Could you check a few things on this model? Use its own coordinates, in mm. Round coordinates to 2 decimals unless told otherwise and drop trailing zeros. Loops run counter-clockwise (first coordinate to the right, second up) from the corner with the lowest first, then second, coordinate; pieces in that order, holes last. Notation, with made-up numbers: (1, -19.5) - (23, -19.5) arc R15 cw to (23, -5.5) - close; hole circle Ø11 at (65, -13). An arc over 180 degrees is marked (long way). Use one line per item in the form item = value.
```python
from build123d import *

# Parameters (mm, degrees)
SKETCH1_R               = 12.5
SKETCH1_R_2             = 3.5
BOSS_EXTRUDE1_DEPTH     = 12
CUT_EXTRUDE1_DEPTH      = 22
CUT_EXTRUDE1_DEPTH_BACK = 22
SKETCH2_R               = 12.5
FILLET2_R               = 1


with BuildPart() as part:
    # Sketch1 → Boss-Extrude1 (new body)
    with BuildSketch(Plane(origin=(0, 0, 0), x_dir=(1, 0, 0), z_dir=(0, 1, 0))):
        with Locations(Location((0, 0, 0), (0, 0, 270))):
            Circle(SKETCH1_R)
        with Locations(Location((0, 0, 0), (0, 0, 270))):
            Circle(SKETCH1_R_2, mode=Mode.SUBTRACT)
    extrude(amount=BOSS_EXTRUDE1_DEPTH)

    # Sketch2 → Cut-Extrude1 (cut, two sides: drawn at the far end of the back side and taken through both)
    with BuildSketch(Plane.XY.offset(-CUT_EXTRUDE1_DEPTH_BACK)):
        with Locations((0, 17)):
            Circle(SKETCH2_R)
    extrude(amount=CUT_EXTRUDE1_DEPTH + CUT_EXTRUDE1_DEPTH_BACK, mode=Mode.SUBTRACT)

    # Fillet2
    fillet2_edges = [part.edges().sort_by_distance(p)[0] for p in [
        (11.456439237, 12, 0),
        (-11.456439237, 12, 0),
    ]]
    fillet(fillet2_edges, radius=FILLET2_R)


solid = part.part
```
1. If we section it at D-D, the plane y = 1: Write out the boundary of the cut face in (x, z).
Solution:
outline = circle Ø25 at (0, 0); hole circle Ø7 at (0, 0)
2. If we section it at C-C, the plane y = 9.5: Write out the boundary of the cut face in (x, z), plus the area to 3 significant figures.
Solution:
outline = (-10, -7.5) - (-10, 7.5) arc R12.5 ccw to start; (10, -7.5) arc R12.5 ccw to (10, 7.5) - close
area = 51.1 mm^2
3. We'd pull the mould along X, two halves only. Please class faces 1 (the face through (-3, 0, 3)), 2 (the face through (2.86, 4.83, 2.6)), 3 (the face through (3.755, 4.583, 11.923)), 4 (the face through (3.47, 2.47, -0.46)): +X half, -X half, draft (parallel to the pull), parting line (faces both ways), or undercut.
Solution:
face_1 = draft
face_2 = undercut
face_3 = parting line
face_4 = undercut
4. If we section it at B-B, the plane z = 0: Write out the boundary of the cut face in (x, y).
Solution:
outline = (-12.5, 0) - (-3.5, 0) - (-3.5, 5) arc R12.5 cw to (-11.2, 11.44) arc R1 ccw to (-12.09, 12) - (-12.5, 12) - close; (3.5, 0) - (12.5, 0) - (12.5, 12) - (12.09, 12) arc R1 ccw to (11.2, 11.44) arc R12.5 cw to (3.5, 5) - close
5. If we section it at A-A, the plane x = 0: Write out the boundary of the cut face in (y, z).
Solution:
outline = (0, -12.5) - (4.5, -12.5) - (4.5, -3.5) - (0, -3.5) - close; (0, 3.5) - (4.5, 3.5) - (4.5, 12.5) - (0, 12.5) - close
6. For P1, Ø10, axis at x = 0.5, z = -6, coming from the +Y side (3 decimals); P2, Ø3, axis at x = 9, y = 3.5, coming from the +Z side; P3, Ø5.5, axis at x = 0, z = 0, coming from the -Y side; P4, Ø2, axis at y = 8.5, z = -4.5, coming from the +X side, each with a flat end and sliding along its axis, tell me the tip position at first contact or that it passes through.
Solution:
P1 = 5.775
P2 = 10
P3 = through
P4 = 12
7. Please list where these lines run through material, in increasing order: line 1 along X through (y, z) = (1.65, 0); line 2 along X through (y, z) = (6.5, 4.75).
Solution:
line_1 = -12.5 to -3.5, 3.5 to 12.5
line_2 = -11.56 to -6.78, 6.78 to 11.56
